The model under review builds one solid part; all positions refer to its coordinate system, in mm. A direction names the side the tool comes from. Give positions to 0.01 mm unless a question says otherwise; leave off trailing zeros. Loops run counter-clockwise (first coordinate to the right, second up) from the corner with the lowest first, then second, coordinate; pieces in that order, holes last. Notation, with made-up numbers: M 1,19 L 49,19 A18 cw 49,37 Z; hole C -40,86.5 d3. An arc over 180 degrees is marked long. Return JSON: item names as keys, results as strings. Group by question number.
```python
from build123d import *

# Parameters (mm, degrees)
CROQUIS1_R              = 0.5
SALIENTE_EXTRUIR1_DEPTH = 18.8
CROQUIS2_R              = 1.5
SALIENTE_EXTRUIR2_DEPTH = 15.3
CORTAR_EXTRUIR1_START   = -8.9
CORTAR_EXTRUIR1_DEPTH   = 8.9


with BuildPart() as part:
    # Croquis1 → Saliente-Extruir1 (new body)
    with BuildSketch(Plane(origin=(0, 0, 0), x_dir=(1, 0, 0), z_dir=(0, 1, 0))):
        with Locations(Location((0, 0, 0), (0, 0, 270))):
            Circle(CROQUIS1_R)
    extrude(amount=SALIENTE_EXTRUIR1_DEPTH)

    # Croquis2 → Saliente-Extruir2 (add)
    with BuildSketch(Plane(origin=(0, 18.8, 0), x_dir=(1, 0, 0), z_dir=(0, 1, 0))):
        with Locations(Location((0, 0, 0), (0, 0, 270))):
            Circle(CROQUIS2_R)
    extrude(amount=SALIENTE_EXTRUIR2_DEPTH)

    # Croquis3 → Cortar-Extruir1 (cut)
    with BuildSketch(Plane(origin=(0, 34.1, 0), x_dir=(1, 0, 0), z_dir=(0, 1, 0)).offset(CORTAR_EXTRUIR1_START)):
        with BuildLine():
            Line((-1.326649916, -0.7), (1.326649916, -0.7))
            ThreePointArc((1.326649916, -0.7), (0, -1.5), (-1.326649916, -0.7))
        make_face()
    extrude(amount=CORTAR_EXTRUIR1_DEPTH, mode=Mode.SUBTRACT)


solid = part.part
```
(1) For probe 1 along Y at (x, z) = (-0.65, -0.45); probe 2 along Y at (x, z) = (1, 1.05); probe 3 along X at (y, z) = (29, -0.7), list the stretches that pass through material, from the lowest coordinate up.
(2) Add section D-D (y = 29). Write out the cut boundary in (x, z).
(3) For faces 1 (the flat face through (0, 18.8, 1)), 2 (the flat face through (0, 30, 0.7)), 3 (the cylindrical face through (-0.9, 26.3, -1.2)), list the 3-axis set-ups (+Z, -Z, +X, -X, +Y, -Y) from which the entire face can be reached by the end or side of a thin tool; tool diameter is ignored.
(4) For pin 1 (1 mm diameter, centred on x = -1, z = 1, fed in from +Y); pin 2 (1.3 mm diameter, centred on x = 0, y = 30, fed in from +Z); pin 3 (1 mm diameter, centred on x = 1, y = 30, fed in from -Z), all flat-tipped, find the tip position at first contact; note any pin that passes through.
(5) Add section A-A (x = 0). Write out the cut boundary in (y, z), and give its area (3 significant figures).
(6) Add section C-C (y = 7). Write out the cut boundary in (x, z).
(7) Add section B-B (z = 0). Write out the cut boundary in (x, y), and give its area (3 significant figures).
Verdict:
{
 "1": {"probe 1": "y = 18.8 to 34.1", "probe 2": "y = 18.8 to 25.2", "probe 3": "x = -1.33 to 1.33"},
 "2": {"outline": "M -1.33,0.7 A1.5 ccw long 1.33,0.7 Z"},
 "3": {"face 1": "-Y", "face 2": "+Z, +X, -X, +Y", "face 3": "+Y, -Y"},
 "4": {"pin 1": "stops at y = 34.1", "pin 2": "stops at z = 0.7", "pin 3": "stops at z = -1.41"},
 "5": {"outline": "M 0,-0.5 L 18.8,-0.5 L 18.8,-1.5 L 34.1,-1.5 L 34.1,0.7 L 25.2,0.7 L 25.2,1.5 L 18.8,1.5 L 18.8,0.5 L 0,0.5 Z", "area": "57.6 mm²"},
 "6": {"outline": "C 0,0 d1"},
 "7": {"outline": "M -1.5,18.8 L -0.5,18.8 L -0.5,0 L 0.5,0 L 0.5,18.8 L 1.5,18.8 L 1.5,34.1 L -1.5,34.1 Z", "area": "64.7 mm²"}
}
